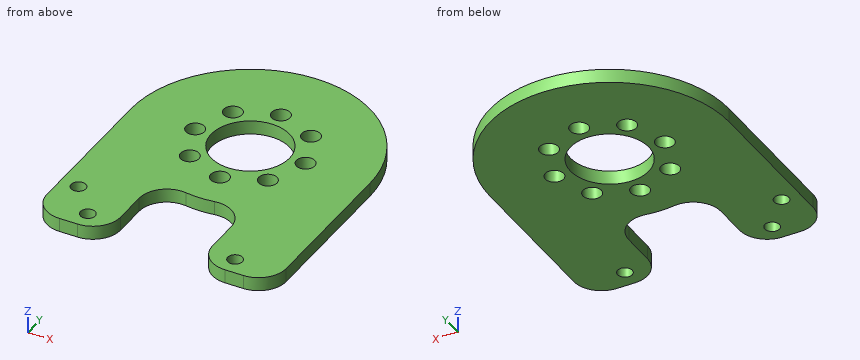
Autodesk Inventor part; units mm, degrees
ref_plane "YZ Plane" through (0, 0, 0) normal (1, 0, 0) x (0, 1, 0)
ref_plane "XZ Plane" through (0, 0, 0) normal (0, 1, 0) x (-1, 0, 0)
ref_plane "XY Plane" through (0, 0, 0) normal (0, 0, 1) x (1, 0, 0)
sketch "スケッチ1" plane through (0, 0, 0) normal (0, 0, 1) x (1, 0, 0)
  line L0 (0, 19.5) -> (26, 19.5)
  line L1 (26, 19.5) -> (26, 0)
  line L2 (26, 0) -> (0, 0)
  line L3 (0, 0) -> (0, 19.5)
  circle A0 centre (13, 19.5) radius 13
  circle A1 centre (13, 19.5) radius 4.25
  circle A2 centre (13, 19.5) radius 6
  circle A3 centre (13, 25.5) radius 1
  circle A4 centre (8.7574, 23.7426) radius 1
  circle A5 centre (7, 19.5) radius 1
  circle A6 centre (8.7574, 15.2574) radius 1
  circle A7 centre (13, 13.5) radius 1
  circle A8 centre (17.2426, 15.2574) radius 1
  circle A9 centre (19, 19.5) radius 1
  circle A10 centre (17.2426, 23.7426) radius 1
  point P0 (0, 19.5)
  dimension "d3" = 12
  dimension "d0" = 19.5
  dimension "d1" = 26
  dimension "d2" = 8.5
  dimension "d4" = 2
  dimension "d7" = 360
extrude "押し出し1" add sketch "スケッチ1" along normal blind 1.5 contours A9 A2 A10 A3 A4 A5 L0 A0 | L0 A0 A5 A2 A6 A7 A8 A9 | A9 A2 A8 A7 A6 A5 L0 A1 | L0 A1 A5 A2 A4 A3 A10 A9 | L1 L2 L3 A0
sketch "スケッチ2" plane through (0, 0, 1.5) normal (0, 0, 1) x (1, 0, 0)
  circle A0 centre (2, 5.5906) radius 0.8
  circle A1 centre (5, 2) radius 0.8
  circle A2 centre (21, 2) radius 0.8
  circle A3 centre (13, 19.5) radius 4.25
  circle A4 centre (13, 19.5) radius 10
  line L0 (0, 0) -> (26, 0)
  line L1 (8, 10.8397) -> (8, 0)
  line L2 (18, 10.8397) -> (18, 0)
  point P0 (2, 0)
  point P1 (24, 0)
  dimension "d14" = 20
  dimension "d16" = 3
  dimension "d17" = 3
extrude "押し出し2" cut sketch "スケッチ2" against normal through all contours A0 | A1 | A2 | A4 L2 L0 L1
fillet "フィレット2" radius 3 6 edges at (0, 0, 0.75) (8, 0, 0.75) (8, 10.8397, 0.75) (18, 10.8397, 0.75) (18, 0, 0.75) (26, 0, 0.75)
properties part number "hipjoint_toleg_upper" material "アルミニウム 6061"
Design review of the part built by this model. Coordinates are the model's own, in mm. Coordinates: 2 decimals unless noted, no trailing zeros. Loops run counter-clockwise (first coordinate to the right, second up) from the corner with the lowest first, then second, coordinate; pieces in that order, holes last.
Q1. We need section D-D on z = 0.8. State how many separate pieces and enclosed holes the cut face has, and give its area (3 significant figures).
Reported:
separate pieces: 1
enclosed holes: 12
area: 585 mm2
Q2. We need section B-B on x = 7. State the section outline as (y, z) points.
Reported:
outline: (0.76, 0) - (18.5, 0) - (18.5, 1.5) - (0.76, 1.5) - close; (20.5, 0) - (31.03, 0) - (31.03, 1.5) - (20.5, 1.5) - close
Q3. For pin 1 (1.6 mm diameter, centred on x = 8.76, y = 23.74, fed in from +Z), flat-tipped, find the tip position at first contact; note if it passes through.
Reported:
pin 1: passes through
Q4. We need section C-C on y = 22. State the section outline as (x, z) points.
Reported:
outline: (0.24, 0) - (9.56, 0) - (9.56, 1.5) - (0.24, 1.5) - close; (16.44, 0) - (25.76, 0) - (25.76, 1.5) - (16.44, 1.5) - close
Q5. We need section A-A on x = 13. State the section outline as (y, z) points.
Reported:
outline: (9.5, 0) - (12.5, 0) - (12.5, 1.5) - (9.5, 1.5) - close; (14.5, 0) - (15.25, 0) - (15.25, 1.5) - (14.5, 1.5) - close; (23.75, 0) - (24.5, 0) - (24.5, 1.5) - (23.75, 1.5) - close; (26.5, 0) - (32.5, 0) - (32.5, 1.5) - (26.5, 1.5) - close
Q6. To check wall thickness, follow line 1 (X direction, y = 19.5, z = 0.5); line 2 (Y direction, x = 13, z = 0.1); line 3 (X direction, y = 20, z = 0.8). State the ranges of each line that lie inside material, in increasing order.
Reported:
line 1: x = 0 to 6, 8 to 8.75, 17.25 to 18, 20 to 26
line 2: y = 9.5 to 12.5, 14.5 to 15.25, 23.75 to 24.5, 26.5 to 32.5
line 3: x = 0.01 to 6.13, 7.87 to 8.78, 17.22 to 18.13, 19.87 to 25.99
